Build history of the part. All positions in model axes, mm. A direction names the side the tool comes from. Round coordinates to 2 decimals unless told otherwise and drop trailing zeros. Write each loop counter-clockwise with the first axis right and the second up, starting at its lowest first coordinate (ties: lowest second). Pieces come first, ordered by that corner, then holes. Notation, with made-up numbers: (-17, 2.5) -> (34, 2.5) arc R27 ccw to (34, 32.5) -> close; hole circle Ø1 at (67, -10). An arc over 180 degrees is marked (long way). Answer in a Markdown table with one row per item.
```python
from build123d import *

# Parameters (mm, degrees)
F0_W      = 30
F0_H      = 55
F1_DEPTH  = 12
F3_W      = 25.3
F3_H      = 14
F4_DEPTH  = 30.001
F5_W      = 7
F5_H      = 7
F6_DEPTH  = 30.001
F7_W      = 7
F7_H      = 7
F8_DEPTH  = 30.001
F10_R     = 2.1
F11_DEPTH = 5.001
F12_R     = 2.1
F13_DEPTH = 5.001


with BuildPart() as f1:
    # F0 (on Top) → F1 (new body)
    with BuildSketch(Plane.XY):
        Rectangle(F0_W, F0_H)
    extrude(amount=F1_DEPTH)

    # F3 (on offset) → F4 (cut, through all)
    with BuildSketch(Plane.YZ.offset(15)):
        Rectangle(F3_W, F3_H)
    extrude(amount=-F4_DEPTH, mode=Mode.SUBTRACT)

    # F5 (on face) → F6 (cut, through all)
    with BuildSketch(Plane.YZ.offset(15)):
        with Locations((-24, 8.5)):
            Rectangle(F5_W, F5_H)
    extrude(amount=-F6_DEPTH, mode=Mode.SUBTRACT)

    # F7 (on face) → F8 (cut, through all)
    with BuildSketch(Plane.YZ.offset(15)):
        with Locations((24, 8.5)):
            Rectangle(F7_W, F7_H)
    extrude(amount=-F8_DEPTH, mode=Mode.SUBTRACT)

    # F10 (on offset) → F11 (cut, through all)
    with BuildSketch(Plane.XY.offset(5)):
        with Locations((-10, 24)):
            Circle(F10_R)
        with Locations((10, 24)):
            Circle(F10_R)
    extrude(amount=-F11_DEPTH, mode=Mode.SUBTRACT)

    # F12 (on face) → F13 (cut, through all)
    with BuildSketch(Plane.XY.offset(5)):
        with Locations((-10, -24)):
            Circle(F12_R)
        with Locations((10, -24)):
            Circle(F12_R)
    extrude(amount=-F13_DEPTH, mode=Mode.SUBTRACT)


solid = f1.part
```
Q1. Saw through at C-C on y = -24. Write the cut outline in (x, z), plus the area to 3 significant figures.
A:
| item | result |
|---|---|
| outline | (-15, 0) -> (-12.1, 0) -> (-12.1, 5) -> (-15, 5) -> close; (-7.9, 0) -> (7.9, 0) -> (7.9, 5) -> (-7.9, 5) -> close; (12.1, 0) -> (15, 0) -> (15, 5) -> (12.1, 5) -> close |
| area | 108 mm² |
Q2. Two-plate mould, pull along X, no slides. Class faces 5 (the flat face through (-15, -0.4, 7.2)), 6 (the flat face through (0, 12.65, 3)), 7 (the cylindrical face through (-11.548, -22.581, 2.535)), 8 (the flat face through (15, -0.4, 7.2)): released by +X, released by -X, zero draft, split by the parting line, or undercut.
A:
| item | result |
|---|---|
| face 5 | released by -X |
| face 6 | zero draft |
| face 7 | undercut |
| face 8 | released by +X |
Q3. Wall check: line 1 (Y direction, x = -10, z = 1.95); line 2 (Y direction, x = -12.5, z = 2); line 3 (Y direction, x = 7, z = 6.75). Give the ranges that are in metal, low to high. Write a range as [from, to].
A:
| item | result |
|---|---|
| line 1 | [-27.5, -26.1], [-21.9, -12.65], [12.65, 21.9], [26.1, 27.5] |
| line 2 | [-27.5, -12.65], [12.65, 27.5] |
| line 3 | [-20.5, -12.65], [12.65, 20.5] |
Q4. Drop flat-ended pins along their axis: P1, Ø3, axis at x = -1.5, z = 9.5, coming from the -Y side; P2, Ø8, axis at x = 10, y = 0.5, coming from the -Z side; P3, Ø4, axis at x = -10, y = 24, coming from the -Z side; P4, Ø2, axis at x = -6.5, y = 25, coming from the +Z side. Give the stop position or say it passes through.
A:
| item | result |
|---|---|
| P1 | y = -20.5 |
| P2 | z = 7 |
| P3 | through |
| P4 | z = 5 |
Q5. Saw through at A-A on z = 2.75. Write the cut outline in (x, y), plus the area to 3 significant figures.
A:
| item | result |
|---|---|
| outline | (-15, -27.5) -> (15, -27.5) -> (15, -12.65) -> (-15, -12.65) -> close; (-15, 12.65) -> (15, 12.65) -> (15, 27.5) -> (-15, 27.5) -> close; hole circle Ø4.2 at (-10, -24); hole circle Ø4.2 at (-10, 24); hole circle Ø4.2 at (10, -24); hole circle Ø4.2 at (10, 24) |
| area | 836 mm² |
Q6. Saw through at D-D on x = -7. Write the cut outline in (y, z), plus the area to 3 significant figures.
A:
| item | result |
|---|---|
| outline | (-27.5, 0) -> (-12.65, 0) -> (-12.65, 7) -> (12.65, 7) -> (12.65, 0) -> (27.5, 0) -> (27.5, 5) -> (20.5, 5) -> (20.5, 12) -> (-20.5, 12) -> (-20.5, 5) -> (-27.5, 5) -> close |
| area | 385 mm² |
Q7. Which spindle directions (+Z, -Z, +X, -X, +Y, -Y) get a long thin tool onto all of the face, cutting with end or side? Do faces 1 (the flat face through (0, -24, 5)), 2 (the flat face through (0, -12.65, 3)), 3 (the flat face through (0, 24, 5)), 4 (the flat face through (0, -20, 0)). Say none if no direction does.
A:
| item | result |
|---|---|
| face 1 | +Z, +X, -X, -Y |
| face 2 | -Z, +X, -X |
| face 3 | +Z, +X, -X, +Y |
| face 4 | -Z, +X, -X, +Y, -Y |
Q8. Saw through at B-B on x = -10. Write the cut outline in (y, z), plus the area to 3 significant figures.
A:
| item | result |
|---|---|
| outline | (-27.5, 0) -> (-26.1, 0) -> (-26.1, 5) -> (-27.5, 5) -> close; (-21.9, 0) -> (-12.65, 0) -> (-12.65, 7) -> (12.65, 7) -> (12.65, 0) -> (21.9, 0) -> (21.9, 5) -> (20.5, 5) -> (20.5, 12) -> (-20.5, 12) -> (-20.5, 5) -> (-21.9, 5) -> close; (26.1, 0) -> (27.5, 0) -> (27.5, 5) -> (26.1, 5) -> close |
| area | 343 mm² |
